Autodesk Inventor part; units mm, degrees
ref_plane "YZ Plane" through (0, 0, 0) normal (1, 0, 0) x (0, 1, 0)
ref_plane "XZ Plane" through (0, 0, 0) normal (0, 1, 0) x (-1, 0, 0)
ref_plane "XY Plane" through (0, 0, 0) normal (0, 0, 1) x (1, 0, 0)
sketch "Эскиз1" plane through (0, 0, 0) normal (0, 1, 0) x (-1, 0, 0)
  line L0 (0, 0) -> (23.1579, 0)
  line L1 (23.1579, 0) -> (23.1579, -40)
  line L2 (23.1579, -40) -> (0, -40)
  line L3 (0, -40) -> (0, 0)
  line L4 (17.9579, -3) -> (12.2807, -3)
  line L5 (12.2807, -3) -> (12.2807, -8.6772)
  line L6 (12.2807, -8.6772) -> (17.9579, -8.6772)
  line L7 (17.9579, -8.6772) -> (17.9579, -3)
  line L8 (17.9579, -10.0807) -> (12.2807, -10.0807)
  line L9 (12.2807, -10.0807) -> (12.2807, -15.7579)
  line L10 (12.2807, -15.7579) -> (17.9579, -15.7579)
  line L11 (17.9579, -15.7579) -> (17.9579, -10.0807)
  line L12 (17.9579, -17.1614) -> (12.2807, -17.1614)
  line L13 (12.2807, -17.1614) -> (12.2807, -22.8386)
  line L14 (12.2807, -22.8386) -> (17.9579, -22.8386)
  line L15 (17.9579, -22.8386) -> (17.9579, -17.1614)
  line L16 (17.9579, -24.2421) -> (12.2807, -24.2421)
  line L17 (12.2807, -24.2421) -> (12.2807, -37)
  line L18 (12.2807, -37) -> (17.9579, -37)
  line L19 (17.9579, -37) -> (17.9579, -24.2421)
  line L20 (10.8772, -24.2421) -> (5.2, -24.2421)
  line L21 (5.2, -24.2421) -> (5.2, -29.9193)
  line L22 (5.2, -29.9193) -> (10.8772, -29.9193)
  line L23 (10.8772, -29.9193) -> (10.8772, -24.2421)
  line L24 (10.8772, -31.3228) -> (5.2, -31.3228)
  line L25 (5.2, -31.3228) -> (5.2, -37)
  line L26 (5.2, -37) -> (10.8772, -37)
  line L27 (10.8772, -37) -> (10.8772, -31.3228)
  line L28 (10.8772, -3) -> (5.2, -3)
  line L29 (5.2, -3) -> (5.2, -22.8386)
  line L30 (5.2, -22.8386) -> (10.8772, -22.8386)
  line L31 (10.8772, -22.8386) -> (10.8772, -3)
  line L32 (15.1193, -8.6772) -> (15.1193, -10.0807)
  line L33 (15.1193, -15.7579) -> (15.1193, -17.1614)
  line L34 (15.1193, -22.8386) -> (15.1193, -24.2421)
  line L35 (8.0386, -22.8386) -> (8.0386, -24.2421)
  line L36 (8.0386, -29.9193) -> (8.0386, -31.3228)
  line L37 (15.1193, -3) -> (15.1193, 0)
  line L38 (15.1193, -37) -> (15.1193, -40)
  line L39 (17.9579, -12.9193) -> (23.1579, -12.9193)
  line L40 (5.2, -12.9193) -> (0, -12.9193)
  line L41 (12.2807, -12.9193) -> (10.8772, -12.9193)
  dimension "d0" = 23.1579
  dimension "d1" = 40
  dimension "d9" = 5.2
  dimension "d21" = 3
extrude "Выдавливание1" add sketch "Эскиз1" along normal blind 0.5 contours L24 L27 L26 L25 | L20 L23 L22 L21 | L4 L7 L6 L5 | L29 L28 L31 L30 | L11 L10 L9 L8 | L18 L17 L16 L19 | L12 L15 L14 L13
sketch "Эскиз2" plane through (0, 0, 0) normal (0, -1, 0) x (1, 0, 0)
  line L0 (-5.2, -22.8386) -> (-10.8772, -22.8386)
  line L1 (-10.8772, -22.8386) -> (-10.8772, -3)
  line L2 (-10.8772, -3) -> (-5.2, -3)
  line L3 (-5.2, -3) -> (-5.2, -22.8386)
  line L4 (-5.2, -31.3228) -> (-5.2, -37)
  line L5 (-5.2, -37) -> (-10.8772, -37)
  line L6 (-10.8772, -37) -> (-10.8772, -31.3228)
  line L7 (-10.8772, -31.3228) -> (-5.2, -31.3228)
  line L8 (-17.9579, -17.1614) -> (-12.2807, -17.1614)
  line L9 (-12.2807, -22.8386) -> (-17.9579, -22.8386)
  line L10 (-17.9579, -22.8386) -> (-17.9579, -17.1614)
  line L11 (-17.9579, -37) -> (-17.9579, -24.2421)
  line L12 (-17.9579, -24.2421) -> (-12.2807, -24.2421)
  line L13 (-12.2807, -37) -> (-17.9579, -37)
  line L14 (-12.2807, -15.7579) -> (-17.9579, -15.7579)
  line L15 (-17.9579, -15.7579) -> (-17.9579, -10.0807)
  line L16 (-17.9579, -10.0807) -> (-12.2807, -10.0807)
  line L17 (-17.9579, -8.6772) -> (-17.9579, -3)
  line L18 (-17.9579, -3) -> (-12.2807, -3)
  line L19 (-12.2807, -8.6772) -> (-17.9579, -8.6772)
  line L20 (-5.2, -24.2421) -> (-5.2, -29.9193)
  line L21 (-5.2, -29.9193) -> (-10.8772, -29.9193)
  line L22 (-10.8772, -29.9193) -> (-10.8772, -24.2421)
  line L23 (-10.8772, -24.2421) -> (-5.2, -24.2421)
  line L24 (-12.2807, -17.1614) -> (-12.2807, -22.8386)
  line L25 (-12.2807, -24.2421) -> (-12.2807, -37)
  line L26 (-12.2807, -10.0807) -> (-12.2807, -15.7579)
  line L27 (-12.2807, -3) -> (-12.2807, -8.6772)
  line L28 (-10.8772, -3) -> (-5.2, -3)
  line L29 (-17.9579, -37) -> (-5.2, -3)
  circle A0 centre (-11.5789, -20) radius 21.35
  dimension "d24" = 42.7
extrude "Выдавливание2" add sketch "Эскиз2" along normal blind 1.5 contours L12 L25 L13 L29 | L29 L11 L12 | L24 L9 L29 | L29 L9 L10 L8 L24 | L0 L1 L29 L3 | L29 L1 L2 | L4 L5 L6 L7 | L14 L15 L16 L26 | L17 L18 L27 L19 | L20 L21 L22 L23 | A0
fillet "Сопряжение1" radius 1 28 edges at (-17.9579, 0.25, -3) (-17.9579, 0.25, -8.6772) (-12.2807, 0.25, -3) (-12.2807, 0.25, -8.6772) (-17.9579, 0.25, -15.7579) (-17.9579, 0.25, -10.0807) (-12.2807, 0.25, -10.0807) (-12.2807, 0.25, -15.7579) (-12.2807, 0.25, -22.8386) (-5.2, 0.25, -29.9193) (-5.2, 0.25, -22.8386) (-5.2, 0.25, -37) (-17.9579, 0.25, -22.8386) (-17.9579, 0.25, -37) (-10.8772, 0.25, -22.8386) (-10.8772, 0.25, -29.9193) (-10.8772, 0.25, -37) (-17.9579, 0.25, -24.2421) (-10.8772, 0.25, -3) (-12.2807, 0.25, -24.2421) (-5.2, 0.25, -24.2421) (-5.2, 0.25, -3) (-10.8772, 0.25, -24.2421) (-17.9579, 0.25, -17.1614) (-12.2807, 0.25, -17.1614) (-12.2807, 0.25, -37) (-10.8772, 0.25, -31.3228) (-5.2, 0.25, -31.3228)
chamfer "Фаска1" distance 1.5 angle 45 1 edges at (-32.9289, 0, -20)
sketch "Эскиз5" plane through (-11.5789, 0, -20) normal (0, 1, 0) x (1, 0, 0)
  circle A0 centre (0, 0) radius 19.85
  circle A1 centre (0, 0) radius 21.35
  circle A2 centre (21.35, 0) radius 1.5
  circle A3 centre (-12.7513, 17.1239) radius 1.5
  circle A4 centre (-12.7513, -17.1239) radius 1.5
  line L0 (28, 0) -> (-19.5959, 20)
  line L1 (28, 0) -> (-19.5959, -20)
  line L2 (-19.5959, 20) -> (-19.5959, -20)
  line L3 (0, 0) -> (-19.5959, 20)
  line L4 (0, 0) -> (-19.5959, -20)
  line L5 (28, 0) -> (0, 0)
  point P0 (11.5789, -20)
  dimension "d28" = 40
  dimension "d29" = 28
extrude "Выдавливание5" cut sketch "Эскиз5" against normal blind 1.5 contours L5 A1 A2 | A2 A1 L5 | A2 L5 A1 | A1 L5 A2 | A3 A1 L0 | L0 A1 A3 | A1 L0 A3 | A4 L1 A1 | A4 A1 L1 | A4 L1 A1 | A3 L0 A1 | A1 L1 A4
equation "\"d0\" = 0.578947 * d1"
properties part number "Лого ШП"
Verification items for the finished model (mm, model axes). A direction names the side the tool comes from. Round coordinates to 2 decimals unless told otherwise and drop trailing zeros.
1. Gauge pin test, flat ends, axial feed: P1, Ø0.6, axis at y = 0, z = -26.5, coming from the -X side; P2, Ø2, axis at x = 5, z = -36, coming from the +Y side (1 decimal); P3, Ø0.6, axis at y = 0.5, z = -20.5, coming from the +X side; P4, Ø0.6, axis at y = 0, z = -16, coming from the +X side. Record the tip position at first contact, or that the pin passes through.
2. Draft check along Z on faces 6 (the cylindrical face through (-17.66, 0.25, -36.71)), 7 (the cylindrical face through (-12.57, 0.25, -8.38)), 8 (the flat face through (-8, 0.5, -27)). Enter one of: +Z half, -Z half, draft (parallel to the pull), parting line (faces both ways), or undercut.
3. Access from +Z, -Z, +X, -X, +Y, -Y to the whole of each face (thin tool, end or side, straight path). Record for faces 1 (the cylindrical face through (-5.501, 0.254, -3.285)), 2 (the cylindrical face through (-10.58, 0.25, -36.71)), 3 (the cylindrical face through (-5.485, 0.254, -36.699)), 4 (the cylindrical face through (-12.58, 0.25, -10.37)), 5 (the cylindrical face through (-17.66, 0.25, -15.47)).
4. Scan lines: L1, parallel to Y at x = -23.5, z = -9.5; L2, parallel to X at y = 0.4, z = -18; L3, parallel to Z at x = 1, y = -1.3. Record each from-to range of solid material in increasing order.
Answer:
1. P1: stops at x = -30.67
1. P2: passes through
1. P3: stops at x = -5.2
1. P4: stops at x = 8.18
2. face 6: -Z half
2. face 7: undercut
2. face 8: draft
3. face 1: +Z, +X, +Y
3. face 2: -Z, +Y
3. face 3: -Z, +X, +Y
3. face 4: +Y
3. face 5: -X, +Y
4. L1: y = -1.5 to 0
4. L2: x = -17.94 to -12.29, -10.88 to -5.2
4. L3: z = -37 to -3
